Source: CAD feature listing. Evaluate the final solid. Frame: model axes, mm. Face numbers are marked on the shaded views. A direction names the side the tool comes from. Give positions to 0.01 mm unless a question says otherwise; leave off trailing zeros. Order: outer loops, then holes, each group sorted by start corner. A loop starts at its lowest first (then second) coordinate and runs counter-clockwise, first axis right, second up.
1) Section A-A, the plane x = 0. Return loops of the section in (y, z).
2) Section C-C, the plane y = -10.5. Return loops of the section in (x, z), plus the area to 3 significant figures.
3) Section B-B, the plane z = 0. Return loops of the section in (x, y), plus the area to 3 significant figures.
4) Draft query along Z for the marked faces 4, 5, 6 and 7. Return one class per face: released by +Z, released by -Z, zero draft, split by the parting line, or undercut.
5) First-contact query: P1, Ø5, axis at x = 14.5, z = 40, coming from the -Y side; P2, Ø1.5, axis at x = -38, y = 12.5, coming from the +Z side; P3, Ø12, axis at x = 25, y = 17, coming from the +Z side. Flat tips, straight axial feed; report the tip coordinate or a pass-through.
6) Material intervals for line 1 (X direction, y = 22, z = -15); line 2 (X direction, y = 31, z = -3.5); line 3 (Y direction, x = -11, z = 26), sorted ascending.
7) Section D-D, the plane y = 5. Return loops of the section in (x, z), plus the area to 3 significant figures.
8) Access query for the marked faces 1, 2 and 3. Directions: +Z, -Z, +X, -X, +Y, -Y. A direction counts if a zero-diameter tool reaches every point of the face in a straight line with its end or side. Return the directions, or none.
```python
from build123d import *

# Parameters (mm, degrees)
EXTRUDE_10_DEPTH      = 35
EXTRUDE_10_DEPTH_BACK = 25
SKETCH_3_R            = 19
SKETCH_3_R_2          = 10


with BuildPart() as part:
    # Эскиз1 → Повернуть-Тонкостенный1 (revolve)
    with BuildSketch(Plane.XY, mode=Mode.PRIVATE) as revolve_1_sk:
        Polygon((19, 0), (43, 0), (50, 21), (52.889577147, 23.332201276), (58.302767501, 25.953006302), (58.738533119, 25.052946123), (53.42847461, 22.482072549), (50.856038751, 20.405838593), (43.72075922, -1), (19, -1), align=None)
    revolve(revolve_1_sk.sketch.rotate(Axis((0, 0, 0), (0, -1, 0)), 90), axis=Axis((0, 0, 0), (0, -1, 0)))

    # Эскиз3 → Вытянуть10 (add, two sides: drawn at the far end of the back side and taken through both)
    with BuildSketch(Plane(origin=(0, 0, 0), x_dir=(1, 0, 0), z_dir=(0, 1, 0)).offset(-EXTRUDE_10_DEPTH_BACK)):
        with Locations(Location((0, 0, 0), (0, 0, 270))):
            Circle(SKETCH_3_R)
        with Locations(Location((0, 0, 0), (0, 0, 270))):
            Circle(SKETCH_3_R_2, mode=Mode.SUBTRACT)
    extrude(amount=EXTRUDE_10_DEPTH + EXTRUDE_10_DEPTH_BACK)


solid = part.part
```
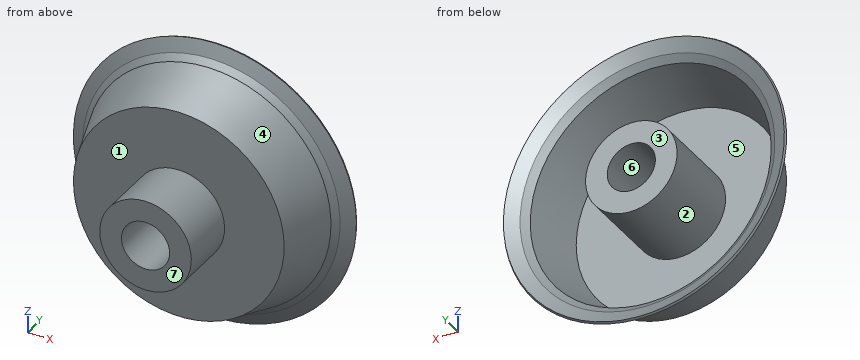
From the geometry:
1. outline: (-25, -19) - (-1, -19) - (-1, -43.72) - (20.41, -50.86) - (22.48, -53.43) - (25.05, -58.74) - (25.95, -58.3) - (23.33, -52.89) - (21, -50) - (0, -43) - (0, -19) - (35, -19) - (35, -10) - (-25, -10) - close; (-25, 10) - (35, 10) - (35, 19) - (0, 19) - (0, 43) - (21, 50) - (23.33, 52.89) - (25.95, 58.3) - (25.05, 58.74) - (22.48, 53.43) - (20.41, 50.86) - (-1, 43.72) - (-1, 19) - (-25, 19) - close
2. outline: circle Ø38 at (0, 0); hole circle Ø20 at (0, 0)
2. area: 820 mm2
3. outline: (-58.74, 25.05) - (-53.43, 22.48) - (-50.86, 20.41) - (-43.72, -1) - (-19, -1) - (-19, -25) - (-10, -25) - (-10, 35) - (-19, 35) - (-19, 0) - (-43, 0) - (-50, 21) - (-52.89, 23.33) - (-58.3, 25.95) - close; (10, -25) - (19, -25) - (19, -1) - (43.72, -1) - (50.86, 20.41) - (53.43, 22.48) - (58.74, 25.05) - (58.3, 25.95) - (52.89, 23.33) - (50, 21) - (43, 0) - (19, 0) - (19, 35) - (10, 35) - close
3. area: 1,190 mm2
4. face 4: split by the parting line
4. face 5: undercut
4. face 6: undercut
4. face 7: zero draft
5. P1: stops at y = -1
5. P2: stops at z = 30.7
5. P3: stops at z = 48.75
6. line 1: x = -50.66 to -48.99, -11.66 to 11.66, 48.99 to 50.66
6. line 2: x = -18.67 to -9.37, 9.37 to 18.67
6. line 3: y = -1 to 0
7. outline: circle Ø91.44 at (0, 0); circle Ø38 at (0, 0); hole circle Ø89.33 at (0, 0); hole circle Ø20 at (0, 0)
7. area: 1,120 mm2
8. face 1: -Y
8. face 2: +Y
8. face 3: +Z, -Z, +X, -X, +Y
